Can you work these out from the model? Positions are in its coordinate system, mm. A direction names the side the tool comes from. Give positions to 0.01 mm unless a question says otherwise; leave off trailing zeros. Order: outer loops, then holes, each group sorted by start corner. A loop starts at its lowest first (then second) coordinate and runs counter-clockwise, first axis right, second up. Notation, with made-up numbers: M 50,-34.75 L 75,-34.75 A25 cw 75,2.25 Z; hole C 79.5,52 d4. An arc over 180 degrees is marked long. Use one line per item in the form item = value. Start each with the question number.
1. I need wall thicknesses on L1, parallel to X at y = -12.5, z = -7; L2, parallel to Y at x = 0, z = -25; L3, parallel to Z at x = 15, y = 10. Which ranges of each line are inside material? Lowest first, please.
2. I want a section at C-C, the plane x = 11. List the corners of the cut face in (y, z) for me.
3. I want a section at D-D, the plane z = 9. List the corners of the cut face in (x, y) for me, and give its area (3 significant figures).
4. I want a section at A-A, the plane x = 0. List the corners of the cut face in (y, z) for me, and give its area (3 significant figures).
5. We'd pull the mould along Y, two halves only. Please class faces 4 (the face through (23.87, 43.61, -23.24)), 5 (the face through (0, 41, -18.95)), 6 (the face through (20.706, 1.183, 15.286)): +Y half, -Y half, draft (parallel to the pull), parting line (faces both ways), or undercut.
6. For faces 1 (the face through (16.142, 2, -2)), 2 (the face through (0, -38, -18.95)), 3 (the face through (-2, -40.847, -23)), which set-ups out of +Z, -Z, +X, -X, +Y, -Y let a thin tool reach every point of the face, with its end or its side?
7. I want a section at B-B, the plane y = -2. List the corners of the cut face in (x, z) for me, and give its area (3 significant figures).
8. Will these pins go through, and if not, where does the flat tip stop? P1, Ø3, axis at x = 0, y = 26.81, coming from the +Z side; P2, Ø3.5, axis at x = 5.5, y = 39.5, coming from the +Z side; P3, Ø1, axis at x = 3, y = 30.5, coming from the +Z side.
```python
from build123d import *

# Parameters (mm, degrees)
F0_R          = 5.370035
F1_DEPTH      = 25.4
F2_R          = 5.08
F3_W          = 32.284736
F3_H          = 39.864631
F4_DEPTH      = 40.848212
F4_DEPTH_BACK = 50.8
F5_R          = 2.592442
F6_DEPTH      = 27.65358


with BuildPart() as f1:
    # F0 (on Right) → F1 (new body, symmetric)
    with BuildSketch(Plane.YZ):
        with BuildLine():
            Line((-8.754894, 16.901342), (-32.144371, -18.949738))
            Line((-32.144371, -18.949738), (34.951739, -18.949738))
            Line((34.951739, -18.949738), (12.647971, 16.698166))
            ThreePointArc((12.647971, 16.698166), (2.002183, 22.661433), (-8.754894, 16.901342))
        make_face()
        with Locations((1.881628, 9.962005)):
            Circle(F0_R, mode=Mode.SUBTRACT)
        Polygon((-32.144371, -18.949738), (-40.847212, -18.949738), (-40.847212, -27.65258), (45.05827, -27.65258), (45.05827, -18.949738), (34.951739, -18.949738), align=None)
    extrude(amount=F1_DEPTH, both=True)

    # F2
    f2_edges = [f1.edges().sort_by_distance(p)[0] for p in [
        (25.4, -40.847212, -23.301159),
        (25.4, 45.05827, -23.301159),
        (0, -32.144371, -18.949738),
        (0, 34.951739, -18.949738),
    ]]
    fillet(f2_edges, radius=F2_R)

    # F3 (on Front) → F4 (cut, two sides)
    with BuildSketch(Plane.XZ) as f4_sk:
        with Locations((0, 3.228473)):
            Rectangle(F3_W, F3_H)
    extrude(amount=F4_DEPTH, mode=Mode.SUBTRACT)
    extrude(f4_sk.sketch, amount=-F4_DEPTH_BACK, mode=Mode.SUBTRACT)

    # F5 (on Top) → F6 (cut, through all)
    with BuildSketch(Plane.XY):
        with Locations((0, 26.810369)):
            Circle(F5_R)
    extrude(amount=-F6_DEPTH, mode=Mode.SUBTRACT)


solid = f1.part
```
Check result:
q1.L1 = -25.4 to -16.14, 16.14 to 25.4
q1.L2 = -40.85 to 24.22, 29.4 to 45.06
q1.L3 = -27.65 to -16.7
q2.outline = M -40.85,-27.65 L 45.06,-27.65 L 45.06,-18.95 L 37.77,-18.95 A5.08 cw 33.55,-16.7 L -30.68,-16.7 A5.08 cw -34.9,-18.95 L -40.85,-18.95 Z
q3.outline = M -25.4,-13.91 L -16.14,-13.91 L -16.14,-3.4 L -25.4,-3.4 Z; M -25.4,7.16 L -16.14,7.16 L -16.14,17.46 L -25.4,17.46 Z; M 16.14,-13.91 L 25.4,-13.91 L 25.4,-3.4 L 16.14,-3.4 Z; M 16.14,7.16 L 25.4,7.16 L 25.4,17.46 L 16.14,17.46 Z
q3.area = 385 mm2
q4.outline = M -40.85,-27.65 L 24.22,-27.65 L 24.22,-16.7 L -30.68,-16.7 A5.08 cw -34.9,-18.95 L -40.85,-18.95 Z; M 29.4,-27.65 L 45.06,-27.65 L 45.06,-18.95 L 37.77,-18.95 A5.08 cw 33.55,-16.7 L 29.4,-16.7 Z
q4.area = 841 mm2
q5.face_4 = +Y half
q5.face_5 = draft
q5.face_6 = undercut
q6.face_1 = +Z, +Y, -Y
q6.face_2 = +Z, +X, -X, -Y
q6.face_3 = +Z, -Z, +X, -X, -Y
q7.outline = M -25.4,-27.65 L 25.4,-27.65 L 25.4,6.25 L 16.14,6.25 L 16.14,-16.7 L -16.14,-16.7 L -16.14,6.25 L -25.4,6.25 Z; M -25.4,13.67 L -16.14,13.67 L -16.14,22.05 L -25.4,22.05 Z; M 16.14,13.67 L 25.4,13.67 L 25.4,22.05 L 16.14,22.05 Z
q7.area = 1,140 mm2
q8.P1 = through
q8.P2 = -18.95
q8.P3 = -16.7
